The drawing under review shows one solid part. Ordinate dimensions are in mm from its lowest x, y, z. A direction names the side the tool comes from. Give positions to 0.01 mm unless a question says otherwise; leave off trailing zeros. Order: outer loops, then holes, each group sorted by start corner. A loop starts at its lowest first (then second) coordinate and runs counter-clockwise, first axis right, second up. Notation, with made-up numbers: (1.25, 66) - (9.25, 66) arc R6 cw to (9.25, 77) - close; hole circle Ø6 at (84, -19). An arc over 180 degrees is marked (long way). Use CSV: the item, a comma, the result in double quotes.
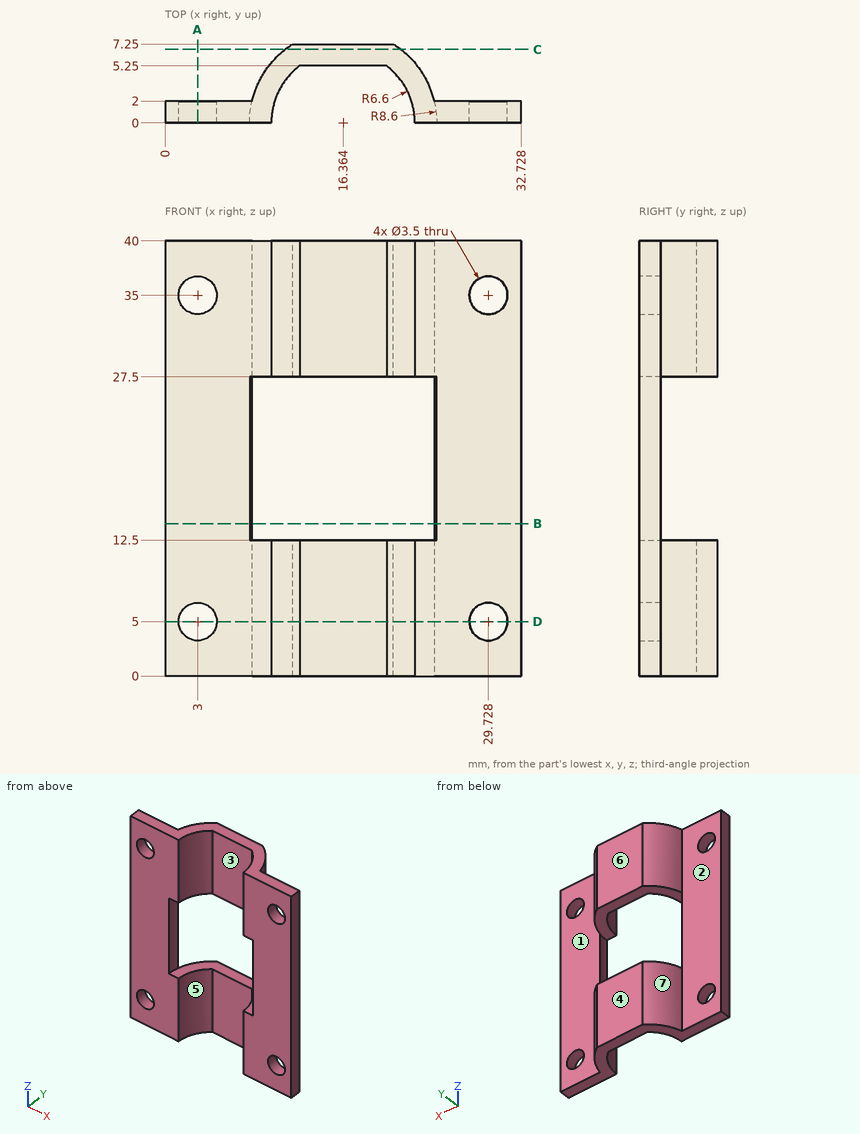
Item 1: Wall thickness on L1, parallel to Z at x = 21.5, y = 6.75; L2, parallel to Y at x = 18.5, z = 11; L3, parallel to X at y = 2.5, z = 11 (1 decimal): over which ranges is each line inside the solid? List them lowest first.
Results list:
L1,"z = 0 to 12.5, 27.5 to 40"
L2,"y = 5.25 to 7.25"
L3,"x = 8.1 to 10.3, 22.5 to 24.6"
Item 2: Take a section at A-A, the plane x = 3. Give the boundary of the cut face in (y, z).
Results list:
outline,"(0, 0) - (2, 0) - (2, 3.25) - (0, 3.25) - close; (0, 6.75) - (2, 6.75) - (2, 33.25) - (0, 33.25) - close; (0, 36.75) - (2, 36.75) - (2, 40) - (0, 40) - close"
Item 3: Take a section at C-C, the plane y = 6.75. Give the boundary of the cut face in (x, z) (1 decimal).
Results list:
outline,"(11, 0) - (21.7, 0) - (21.7, 12.5) - (11, 12.5) - close; (11, 27.5) - (21.7, 27.5) - (21.7, 40) - (11, 40) - close"
Item 4: Mouldability with a two-part tool opening along X and no side actions: class the marked faces 5, 6 and 7 as pulls with the +X half, pulls with the -X half, needs draft (parallel to the pull), parting line crosses it, or undercut.
Results list:
face 5,"undercut"
face 6,"needs draft"
face 7,"pulls with the -X half"
Item 5: Clearance check with flat-ended pins moving along their axes: pin 1 (2.5 mm diameter, centred on x = 18, z = 35.5, fed in from -Y); pin 2 (6.5 mm diameter, centred on x = 15, z = 7.5, fed in from -Y); pin 3 (1 mm diameter, centred on x = 6.5, y = 1.5, fed in from -Z); pin 4 (8 mm diameter, centred on x = 15, z = 5.5, fed in from -Y) (1 decimal). State where each tip first meets the part, or that it passes through.
Results list:
pin 1,"stops at y = 5.25"
pin 2,"stops at y = 4.72"
pin 3,"stops at z = 0"
pin 4,"stops at y = 3.8"
Item 6: Tool access review of the marked faces 1, 2, 3 and 4: name each direction out of +Z, -Z, +X, -X, +Y, -Y from which nothing blocks a thin tool from reaching the whole face with its end or side.
Results list:
face 1,"+Z, -Z, +X, +Y"
face 2,"+Z, -Z, -X, +Y"
face 3,"+Z, -Z, -Y"
face 4,"+Z, -Z, +X, -X, +Y"
Item 7: Take a section at D-D, the plane z = 5. State how many separate pieces and enclosed holes the cut face has.
Results list:
separate pieces,"3"
enclosed holes,"0"
Item 8: Take a section at B-B, the plane z = 14. Give the boundary of the cut face in (x, y) (1 decimal).
Results list:
outline,"(0, 0) - (7.8, 0) arc R8.6 cw to (8, 2) - (0, 2) - close; (24.7, 2) arc R8.6 cw to (25, 0) - (32.7, 0) - (32.7, 2) - close"
